The listing builds one solid part. Answer for the finished solid, in the listing's coordinates (mm). A direction names the side the tool comes from. Give positions to 0.01 mm unless a question says otherwise; leave off trailing zeros. Answer as a JSON object with one key per item and string values. Group by question number.
Q1. A cutting plane is placed at A-A, the plane y = -1. Count the separate pieces of the cut face and the enclosed holes in it, and give its area (3 significant figures).
Q2. Given pin 1 (7.5 mm diameter, centred on y = 1.5, z = -0.5, fed in from +X); pin 2 (2 mm diameter, centred on y = -1.5, z = 3, fed in from +X); pin 3 (1.5 mm diameter, centred on x = -19.5, z = -9.5, fed in from +Y); pin 4 (6 mm diameter, centred on x = -22, y = -5.5, fed in from +Z), each flat-ended and moving along its own axis, determine where each tip first touches the part or whether it passes through.
Q3. For faces 5 (the face through (-12.82, -3.91, -6.54)), 6 (the face through (0, 4, 4)), determine the directions among +Z, -Z, +X, -X, +Y, -Y from which every point of the face is accessible in a straight line to the end or side of a thin tool.
Q4. Consider line 1 (Y direction, x = -9.5, z = -5.5); line 2 (Z direction, x = -12.7, y = 12.5) (3 decimals); line 3 (X direction, y = -11, z = 14.5). Determine where each line is inside the solid, lowest interval first.
Q5. The mould has two halves that part along X. Classify faces 1 (the face through (-12.7, 0, 0)), 2 (the face through (-5.074, 11.957, 3.162)), 3 (the face through (-5.074, -8.717, 8.774)), 4 (the face through (-6.26, -2.9, 3.78)): released by +X, released by -X, zero draft, split by the parting line, or undercut.
from build123d import *

# Parameters (mm, degrees)
SKETCH3_R          = 4.7625
CUT_EXTRUDE1_DEPTH = 12.7
SKETCH4_R          = 8.255
CUT_EXTRUDE2_DEPTH = 21.844
CIRPATTERN1_COUNT  = 3


with BuildPart() as part:
    # Sketch2 → Revolve1 (revolve)
    with BuildSketch(Plane.XY):
        with BuildLine():
            Line((0, 0), (-38.1, 0))
            add(Edge.make_bspline(
                [(0, 19.05), (-14.199031657, 19.05), (-38.1, 16.933744176), (-38.1, 0)],
                knots=[0, 0, 0, 0, 1, 1, 1, 1], degree=3))
            Line((0, 19.05), (0, 0))
        make_face()
    revolve(axis=Axis((0, 0, 0), (-1, 0, 0)))

    # Sketch3 → Cut-Extrude1 (cut)
    with BuildSketch(Plane(origin=(0, 0, 0), x_dir=(0, 0, -1), z_dir=(1, 0, 0))):
        Circle(SKETCH3_R)
    extrude(amount=-CUT_EXTRUDE1_DEPTH, mode=Mode.SUBTRACT)

    # Sketch4 → Cut-Extrude2 (cut)
    with BuildSketch(Plane(origin=(0, 7.62, 0), x_dir=(1, 0, 0), z_dir=(0, 1, 0))):
        with Locations((-12.7, 0)):
            Circle(SKETCH4_R)
    cut_extrude2 = extrude(amount=CUT_EXTRUDE2_DEPTH, mode=Mode.SUBTRACT)

    # CirPattern1: Cut-Extrude2 ×3 about axis
    cirpattern1_axis = Axis((0, 0, 0), (1, 0, 0))
    for i in range(1, CIRPATTERN1_COUNT):
        add(cut_extrude2.rotate(cirpattern1_axis, i * 360 / CIRPATTERN1_COUNT), mode=Mode.SUBTRACT)


solid = part.part
Reply:
{
 "1": {"separate pieces": "1", "enclosed holes": "2", "area": "862 mm^2"},
 "2": {"pin 1": "stops at x = 0", "pin 2": "stops at x = -12.7", "pin 3": "stops at y = 14.88", "pin 4": "stops at z = 16.81"},
 "3": {"face 5": "none", "face 6": "+Z, -Z, +X, +Y, -Y"},
 "4": {"line 1": "y = -17.86 to -11.96, -5.71 to 7.62", "line 2": "z = -13.459 to -8.255, 8.255 to 13.459", "line 3": "x = -4.77 to 0"},
 "5": {"face 1": "released by +X", "face 2": "undercut", "face 3": "undercut", "face 4": "zero draft"}
}
